Model file for the job. Use its own axes, mm. A direction names the side the tool comes from. Give positions to 0.01 mm unless a question says otherwise; leave off trailing zeros. Write each loop counter-clockwise with the first axis right and the second up, starting at its lowest first coordinate (ties: lowest second). Pieces come first, ordered by that corner, then holes.
Autodesk Inventor part; units mm, degrees
ref_plane "YZ Plane" through (0, 0, 0) normal (1, 0, 0) x (0, 1, 0)
ref_plane "XZ Plane" through (0, 0, 0) normal (0, 1, 0) x (-1, 0, 0)
ref_plane "XY Plane" through (0, 0, 0) normal (0, 0, 1) x (1, 0, 0)
sketch "Sketch1" plane through (0, 0, 0) normal (0, 0, 1) x (1, 0, 0)
  line L0 (-8, 24) -> (8, 24)
  line L1 (8, 24) -> (8, -24)
  line L2 (8, -24) -> (-8, -24)
  line L3 (-8, -24) -> (-8, 24)
  point P0 (0, 0)
  dimension "d0" = 16
  dimension "d1" = 48
  dimension "d2" = 8
  dimension "d3" = 24
extrude "Extrusion1" add sketch "Sketch1" along normal blind 9.6
shell "Shell1" thickness 1.5 removed faces 1 at (-2.6667, 8, 0)
sketch "Sketch2" plane through (0, 0, 9.6) normal (0, 0, 1) x (1, 0, 0)
  circle A0 centre (4, -20) radius 2.5
  line L0 (8, 24) -> (8, -24)
  line L1 (8, -24) -> (-8, -24)
  dimension "d7" = 5
  dimension "d10" = 4
  dimension "d11" = 4
extrude "Extrusion2" add sketch "Sketch2" along normal blind 1.6
sketch "Sketch3" plane through (6.5, -22.5, 8.1) normal (0, 0, -1) x (-1, 0, 0)
  circle A0 centre (2.5, 2.5) radius 2.5
  circle A1 centre (2.5, 2.5) radius 1.2
  point P0 (6.5, 22.5)
  dimension "d18" = 2.4
extrude "Extrusion3" cut sketch "Sketch3" against normal blind 1.6 contours A1
pattern_linear "Rectangular Pattern1" count 6 spacing 8 along (0, 1, 0) count 2 spacing 8 along (-1, 0, 0) of "Extrusion2", "Extrusion3"
sketch "Sketch4" plane through (6.5, -22.5, 8.1) normal (0, 0, -1) x (-1, 0, 0)
  circle A0 centre (2.5, 10.5) radius 1.2
  circle A1 centre (2.5, 2.5) radius 1.2
  line L0 (0, 45) -> (0, 0)
  line L1 (0, 0) -> (13, 0)
  circle A2 centre (6.5, 6.5) radius 3.15
  circle A3 centre (6.5, 6.5) radius 2.5
  point P0 (6.5, 22.5)
  dimension "d21" = 6.5
  dimension "d22" = 6.5
  dimension "d23" = 10.5
  dimension "d24" = 2.5
  dimension "d25" = 5
  dimension "d26" = 6.3
extrude "Extrusion4" add sketch "Sketch4" along normal up to surface (8.1 mm away) contours A2
pattern_linear "Rectangular Pattern2" count 5 spacing 8 along (0, 1, 0) of "Extrusion4"
equation "\"d0\" = 0.8 * WIDTH"
equation "\"d1\" = 0.8 * LENGTH"
equation "\"d21\" = 0.5 * d23 + 0.5 * d24"
equation "\"d22\" = d21"
equation "\"WIDTH\" = 2"
properties part number "2456" material "Steel"
1. Probe probe 1 along X at (y, z) = (-12, 7.25); probe 2 along X at (y, z) = (-17, 5); probe 3 along Y at (x, z) = (3.5, 6.5). List the from-to ranges inside material, lowest first.
Calculated:
probe 1: x = -8 to -6.5, 6.5 to 8
probe 2: x = -8 to -6.5, -2.99 to -2.29, 2.29 to 2.99, 6.5 to 8
probe 3: y = -24 to -22.5, 22.5 to 24
2. Slice it at C-C, the plane y = 4. Write the cut outline in (x, z), and give its area (3 significant figures).
Calculated:
outline: (-8, 0) - (-6.5, 0) - (-6.5, 8.1) - (-5.2, 8.1) - (-5.2, 9.7) - (-2.8, 9.7) - (-2.8, 8.1) - (2.8, 8.1) - (2.8, 9.7) - (5.2, 9.7) - (5.2, 8.1) - (6.5, 8.1) - (6.5, 0) - (8, 0) - (8, 9.6) - (6.5, 9.6) - (6.5, 11.2) - (1.5, 11.2) - (1.5, 9.6) - (-1.5, 9.6) - (-1.5, 11.2) - (-6.5, 11.2) - (-6.5, 9.6) - (-8, 9.6) - close
area: 56.6 mm2
3. Pull direction X, two halves, no side cores. Call faces 4 (the flat face through (-8, 0, 5)), 5 (the cylindrical face through (0.54, 18.44, 4.11)), 6 (the flat face through (-4, -20, 11.2)): +X half, -X half, draft (parallel to the pull), parting line (faces both ways), or undercut.
Calculated:
face 4: -X half
face 5: undercut
face 6: draft
4. Pin check, flat tips, straight feed: P1, Ø2, axis at x = -4, y = -12, coming from the -Z side; P2, Ø4, axis at x = -5, y = -9, coming from the -Z side; P3, Ø3, axis at x = -4, y = 12, coming from the -Z side; P4, Ø1, axis at x = -2.5, y = -9, coming from the +Z side. Stop position of each tip, or through.
Calculated:
P1: stops at z = 9.7
P2: stops at z = 0
P3: stops at z = 8.1
P4: stops at z = 9.6
5. Slice it at A-A, the plane z = 6.75. State how many separate pieces and enclosed holes the cut face has, and give its area (3 significant figures).
Calculated:
separate pieces: 6
enclosed holes: 6
area: 241 mm2
6. Which spindle directions (+Z, -Z, +X, -X, +Y, -Y) get a long thin tool onto all of the face, cutting with end or side? Do faces 1 (the cylindrical face through (0.54, 2.44, 4.11)), 2 (the flat face through (0, -24, 5)), 3 (the cylindrical face through (3.46, -9.56, 10.39)). Say none if no direction does.
Calculated:
face 1: -Z
face 2: +Z, -Z, +X, -X, -Y
face 3: +Z
7. Slice it at D-D, the plane y = -15. Write the cut outline in (x, z).
Calculated:
outline: (-8, 0) - (-6.5, 0) - (-6.5, 8.1) - (-2.99, 8.1) - (-2.99, 0) - (-2.29, 0) - (-2.29, 8.1) - (2.29, 8.1) - (2.29, 0) - (2.99, 0) - (2.99, 8.1) - (6.5, 8.1) - (6.5, 0) - (8, 0) - (8, 9.6) - (-8, 9.6) - close
